Can you work these out from the model? Positions are in its coordinate system, mm. A direction names the side the tool comes from. Give positions to 0.01 mm unless a question says otherwise; leave off trailing zeros. Order: outer loops, then holes, each group sorted by start corner. A loop starts at its lowest first (then second) coordinate and runs counter-clockwise, first axis right, second up. Notation, with made-up numbers: (8, -20) - (61, -20) arc R26 cw to (61, 18) - close; hole circle Ø10 at (52, 12). An arc over 180 degrees is marked (long way). Answer as a JSON object with one key per item and string values.
```python
from build123d import *

# Parameters (mm, degrees)
BOSS_EXTRUDE2_DEPTH            = 3.81
SKETCH3_R                      = 6.35
CUT_EXTRUDE1_DEPTH             = 12.7
SKETCH4_R                      = 6.35
SKETCH4_R_2                    = 6.223
BOSS_EXTRUDE3_DEPTH            = 2.54
CUT_EXTRUDE5_DEPTH             = 8.89
SKETCH8_W                      = 3.175
SKETCH8_H                      = 3.175
CUT_EXTRUDE6_DEPTH             = 2.54
F_1_16_0_0625_DIAMETER_HOLE2_D = 1.5875
FILLET1_R                      = 2.54
FILLET2_R                      = 0.254
FILLET3_R                      = 0.254


with BuildPart() as part:
    # Sketch1 → Boss-Extrude2 (new, symmetric)
    with BuildSketch(Plane.XY):
        with BuildLine():
            Line((-1.27, 11.636686539), (1.27, 11.636686539))
            ThreePointArc((1.27, 11.636686539), (1.707470415, 8.829743837), (3.008049424, 6.30411482))
            ThreePointArc((3.008049424, 6.30411482), (3.4925, 6.049187445), (3.95549887, 5.757104627))
            ThreePointArc((3.95549887, 5.757104627), (6.793047264, 5.893584674), (9.442666158, 6.918195532))
            Line((9.442666158, 6.918195532), (10.712666158, 4.718491007))
            ThreePointArc((10.712666158, 4.718491007), (8.50051768, 2.936159163), (6.963548294, 0.547010193))
            ThreePointArc((6.963548294, 0.547010193), (6.985, 0), (6.963548294, -0.547010193))
            ThreePointArc((6.963548294, -0.547010193), (8.50051768, -2.936159163), (10.712666158, -4.718491007))
            Line((10.712666158, -4.718491007), (9.442666158, -6.918195532))
            ThreePointArc((9.442666158, -6.918195532), (6.793047264, -5.893584674), (3.95549887, -5.757104627))
            ThreePointArc((3.95549887, -5.757104627), (3.4925, -6.049187445), (3.008049424, -6.30411482))
            ThreePointArc((3.008049424, -6.30411482), (1.707470415, -8.829743837), (1.27, -11.636686539))
            Line((1.27, -11.636686539), (-1.27, -11.636686539))
            ThreePointArc((-1.27, -11.636686539), (-1.707470415, -8.829743837), (-3.008049424, -6.30411482))
            ThreePointArc((-3.008049424, -6.30411482), (-3.4925, -6.049187445), (-3.95549887, -5.757104627))
            ThreePointArc((-3.95549887, -5.757104627), (-6.793047264, -5.893584674), (-9.442666158, -6.918195532))
            Line((-9.442666158, -6.918195532), (-9.950635894, -6.038366142))
            Line((-9.950635894, -6.038366142), (-5.86342506, -3.796112691))
            ThreePointArc((-5.86342506, -3.796112691), (-5.99767393, -3.580241951), (-6.123978846, -3.359629161))
            Line((-6.123978846, -3.359629161), (-10.204696423, -5.598320397))
            Line((-10.204696423, -5.598320397), (-10.712666158, -4.718491007))
            ThreePointArc((-10.712666158, -4.718491007), (-8.50051768, -2.936159163), (-6.963548294, -0.547010193))
            ThreePointArc((-6.963548294, -0.547010193), (-6.985, 0), (-6.963548294, 0.547010193))
            ThreePointArc((-6.963548294, 0.547010193), (-8.50051768, 2.936159163), (-10.712666158, 4.718491007))
            Line((-10.712666158, 4.718491007), (-9.442666158, 6.918195532))
            ThreePointArc((-9.442666158, 6.918195532), (-6.793047264, 5.893584674), (-3.95549887, 5.757104627))
            ThreePointArc((-3.95549887, 5.757104627), (-3.4925, 6.049187445), (-3.008049424, 6.30411482))
            ThreePointArc((-3.008049424, 6.30411482), (-1.707470415, 8.829743837), (-1.27, 11.636686539))
        make_face()
    extrude(amount=BOSS_EXTRUDE2_DEPTH, both=True)

    # Sketch3 → Cut-Extrude1 (cut)
    with BuildSketch(Plane.XY.offset(3.81)):
        Circle(SKETCH3_R)
    extrude(amount=-CUT_EXTRUDE1_DEPTH, mode=Mode.SUBTRACT)

    # Sketch4 → Boss-Extrude3 (add, symmetric)
    with BuildSketch(Plane.XY):
        Circle(SKETCH4_R)
        Circle(SKETCH4_R_2, mode=Mode.SUBTRACT)
    extrude(amount=BOSS_EXTRUDE3_DEPTH, both=True)

    # Sketch7 → Cut-Extrude5 (cut)
    with BuildSketch(Plane(origin=(0, 0, -3.81), x_dir=(-1, 0, 0), z_dir=(0, 0, -1))):
        Polygon((6.123978846, -3.359629161), (4.840992118, -2.655779632), (4.596655451, -3.101159912), (5.86342506, -3.796112691), (6.123978846, -3.939053109), (6.368315512, -3.493672829), align=None)
    extrude(amount=-CUT_EXTRUDE5_DEPTH, mode=Mode.SUBTRACT)

    # Sketch8 → Cut-Extrude6 (cut)
    with BuildSketch(Plane(origin=(0.733009999, -1.336140839, 0), x_dir=(-0.8767328340240498, -0.4809776894453194, 0), z_dir=(0.4809776894453194, -0.8767328340240498, 0))):
        with Locations((10.018693164, 0)):
            Rectangle(SKETCH8_W, SKETCH8_H)
    cut_extrude6 = extrude(amount=CUT_EXTRUDE6_DEPTH, mode=Mode.SUBTRACT)

    # Mirror2: Cut-Extrude6 across plane
    add(cut_extrude6.mirror(Plane(origin=(0.122168333, -0.22269014, 0), x_dir=(0, 0, 1), z_dir=(0.4809776894453193, -0.8767328340240499, 0))), mode=Mode.SUBTRACT)

    # 1/16 (0.0625) Diameter Hole2 (through all)
    with Locations(Plane(origin=(0.733009999, -1.336140839, 0), x_dir=(-0.8767328340240498, -0.4809776894453194, 0), z_dir=(0.4809776894453194, -0.8767328340240498, 0))):
        with Locations((9.767262648, 0)):
            Hole(F_1_16_0_0625_DIAMETER_HOLE2_D / 2)

    # Fillet1
    fillet1_edges = [part.edges().sort_by_distance(p)[0] for p in [
        (-6.963548294, 0.547010193, 0),
        (-6.963548294, -0.547010193, 0),
        (-3.95549887, -5.757104627, 0),
        (-3.008049424, -6.30411482, 0),
        (3.008049424, -6.30411482, 0),
        (3.95549887, -5.757104627, 0),
        (6.963548294, -0.547010193, 0),
        (6.963548294, 0.547010193, 0),
        (3.95549887, 5.757104627, 0),
        (3.008049424, 6.30411482, 0),
        (-3.008049424, 6.30411482, 0),
        (-3.95549887, 5.757104627, 0),
    ]]
    fillet(fillet1_edges, radius=FILLET1_R)

    # Fillet2
    # the kernel refuses this fillet: 0.254 mm, written as the material it takes off along each edge
    with BuildSketch(Plane(origin=(-10.204696423, -5.598320397, 4.431287546), x_dir=(-0.4999999999999982, 0.8660254037844397, 0), z_dir=(0, 0, -1))) as fillet2_piece_1:
        with BuildLine():
            CenterArc((FILLET2_R * 0.978405584541, FILLET2_R), FILLET2_R, 181.250724062, 88.749275938)
            Line((-FILLET2_R * 0.0213561667787, FILLET2_R * 0.978172480701), (0, 0))
            Line((0, 0), (FILLET2_R * 0.978405584541, 0))
        make_face()
    extrude(amount=8.862575092, mode=Mode.SUBTRACT)
    with BuildSketch(Plane(origin=(-9.442666158, -6.918195532, 4.439805222), x_dir=(-0.5000000000000004, 0.8660254037844385, 0), z_dir=(0, 0, -1)), Plane(origin=(1.27, -11.636686539, 4.439805222), x_dir=(-1, 0, 0), z_dir=(0, 0, -1))) as fillet2_piece_2:
        with BuildLine():
            CenterArc((0.251922089, 0.254), FILLET2_R, 181.265494036, 88.734505964)
            ThreePointArc((-0.002015959, 0.248390349), (-0.000140392, 0.124202216), (0, 0))
            Line((0, 0), (0.251922089, 0))
        make_face()
    extrude(amount=8.879610443, mode=Mode.SUBTRACT)
    with BuildSketch(Plane(origin=(-1.27, -11.636686539, 4.439805222), x_dir=(-0.008115823056968435, 0.9999670661657352, 0), z_dir=(0, 0, -1)), Plane(origin=(-10.712666158, -4.718491007, 4.439805222), x_dir=(0.8619389707188404, 0.5070120420228162, 0), z_dir=(0, 0, -1))) as fillet2_piece_3:
        with BuildLine():
            CenterArc((0.25194708, 0.253975211), FILLET2_R, 180.465007513, 88.734505964)
            Line((-0.002044555, 0.251913792), (0, 0))
            ThreePointArc((0, 0), (0.124199265, 0.000867616), (0.248398529, 0))
        make_face()
    extrude(amount=8.879610443, mode=Mode.SUBTRACT)
    with BuildSketch(Plane(origin=(10.712666158, 4.718491007, 4.439805222), x_dir=(-0.5000000000000051, 0.8660254037844357, 0), z_dir=(0, 0, -1)), Plane(origin=(9.442666158, -6.918195532, 4.439805222), x_dir=(0.5000000000000029, 0.866025403784437, 0), z_dir=(0, 0, -1)), Plane(origin=(1.27, 11.636686539, 4.439805222), x_dir=(-1, 0, 0), z_dir=(0, 0, -1))) as fillet2_piece_4:
        with BuildLine():
            CenterArc((0.251922089, -0.254), FILLET2_R, 90, 88.734505964)
            ThreePointArc((-0.002015959, -0.248390349), (-0.000140392, -0.124202216), (0, 0))
            Line((0, 0), (0.251922089, 0))
        make_face()
    extrude(amount=8.879610443, mode=Mode.SUBTRACT)
    with BuildSketch(Plane(origin=(9.442666158, 6.918195532, 4.439805222), x_dir=(-0.8700547937758036, -0.4929550241429169, 0), z_dir=(0, 0, -1)), Plane(origin=(10.712666158, -4.718491007, 4.439805222), x_dir=(-0.8619389707188434, 0.5070120420228111, 0), z_dir=(0, 0, -1)), Plane(origin=(-9.442666158, 6.918195532, -4.439805222), x_dir=(0.8700547937757986, -0.4929550241429255, 0), z_dir=(0, 0, 1)), Plane(origin=(-1.27, 11.636686539, 4.439805222), x_dir=(-0.008115823056962063, -0.9999670661657353, 0), z_dir=(0, 0, -1))) as fillet2_piece_5:
        with BuildLine():
            CenterArc((0.25194708, -0.253975211), FILLET2_R, 90.800486523, 88.734505964)
            Line((-0.002044555, -0.251913792), (0, 0))
            ThreePointArc((0, 0), (0.124199265, -0.000867616), (0.248398529, 0))
        make_face()
    extrude(amount=8.879610443, mode=Mode.SUBTRACT)
    with BuildSketch(Plane(origin=(-9.950635894, -6.038366142, 4.459015102), x_dir=(0.8767328340240489, 0.48097768944532077, 0), z_dir=(0, 0, -1))) as fillet2_piece_6:
        with BuildLine():
            CenterArc((FILLET2_R * 1.02207102637, FILLET2_R), FILLET2_R, 178.749275938, 91.250724062)
            Line((FILLET2_R * 0.0223092750529, FILLET2_R * 1.0218275193), (0, 0))
            Line((0, 0), (FILLET2_R * 1.02207102637, 0))
        make_face()
    extrude(amount=8.918030203, mode=Mode.SUBTRACT)

    # Fillet3
    fillet3_edges = [part.edges().sort_by_distance(p)[0] for p in [
        (-10.712666158, 4.718491007, 0),
    ]]
    fillet(fillet3_edges, radius=FILLET3_R)


solid = part.part
```
Q1. Which directions (+Z, -Z, +X, -X, +Y, -Y) give clear straight access to the entire face, cutting with the end or side of a thin tool? Please do faces 4 (the face through (-5.97, -5.76, 0.05)), 5 (the face through (-8.014, -2.346, 0.053)), 6 (the face through (-7.293, -5.739, -0.728)), 7 (the face through (-8.7, -3.4, -1.588)), 8 (the face through (-7.068, 5.956, 0.053)).
Recorded:
{"face 4": "+Z, -Z, -Y", "face 5": "+Z, -Z, -X", "face 6": "-Y", "face 7": "-X", "face 8": "+Z, -Z, +Y"}
Q2. I need wall thicknesses on L1, parallel to Y at x = 0, z = 1.2; L2, parallel to Y at x = 0, z = 3.3; L3, parallel to X at y = 0, z = -3.15 (3 decimals). Which ranges of each line are inside material? Lowest first, please.
Recorded:
{"L1": "y = -11.64 to -6.22, 6.22 to 11.64", "L2": "y = -11.64 to -6.35, 6.35 to 11.64", "L3": "x = -6.985 to -6.35, 6.35 to 6.985"}
Q3. If we section it at B-B, the plane y = 2.75: Please give me the cut outline in (x, z), then the cut area to 3 significant figures.
Recorded:
{"outline": "(-8.34, -3.81) - (-5.72, -3.81) - (-5.72, -2.54) - (-5.58, -2.54) - (-5.58, 2.54) - (-5.72, 2.54) - (-5.72, 3.81) - (-8.34, 3.81) - close; (5.58, -2.54) - (5.72, -2.54) - (5.72, -3.81) - (8.34, -3.81) - (8.34, 3.81) - (5.72, 3.81) - (5.72, 2.54) - (5.58, 2.54) - close", "area": "41.3 mm^2"}
Q4. If we section it at A-A, the plane x = 0: Please give me the cut outline in (y, z).
Recorded:
{"outline": "(-11.64, -3.81) - (-6.35, -3.81) - (-6.35, -2.54) - (-6.22, -2.54) - (-6.22, 2.54) - (-6.35, 2.54) - (-6.35, 3.81) - (-11.64, 3.81) - close; (6.22, -2.54) - (6.35, -2.54) - (6.35, -3.81) - (11.64, -3.81) - (11.64, 3.81) - (6.35, 3.81) - (6.35, 2.54) - (6.22, 2.54) - close"}
Q5. We'd pull the mould along X, two halves only. Please class faces 1 (the face through (-8.647, 3.095, 0.053)), 2 (the face through (7, 5.94, 0.05)), 3 (the face through (1.64, -9.04, 0.05)): released by +X, released by -X, zero draft, split by the parting line, or undercut.
Recorded:
{"face 1": "released by -X", "face 2": "undercut", "face 3": "released by +X"}
Q6. If we section it at C-C, the plane y = -7.75: Please give me the cut outline in (x, z).
Recorded:
{"outline": "(-2.14, -3.81) - (2.14, -3.81) - (2.14, 3.81) - (-2.14, 3.81) - close"}
Q7. I'm going to push flat-ended pins straight in: pin 1 Ø4 at (x, y) = (-0.5, 6) entering from +Z; pin 2 Ø3 at (y, z) = (1.5, -3) entering from -X; pin 3 Ø1.5 at (y, z) = (8.5, -2.5) entering from -X; pin 4 Ø1.5 at (y, z) = (-8, -2) entering from -X. Where does each tip first touch, or does it pass through?
Recorded:
{"pin 1": "stops at z = 3.81", "pin 2": "stops at x = -8.56", "pin 3": "stops at x = -2.14", "pin 4": "stops at x = -2.4"}
